Design review of the part shown in the three views and the two pictorial views. Dimensions are in mm from the part's minimum x, y and z. Give positions to 0.01 mm unless a question says otherwise; leave off trailing zeros. Order: outer loops, then holes, each group sorted by start corner. A loop starts at its lowest first (then second) coordinate and runs counter-clockwise, first axis right, second up. Notation, with made-up numbers: (88, -26) - (107, -26) arc R20 ccw to (107, -22) - close; hole circle Ø9 at (54.5, -26.75). An arc over 180 degrees is marked (long way). Put each result on its own line as item: value. Start each with the question number.
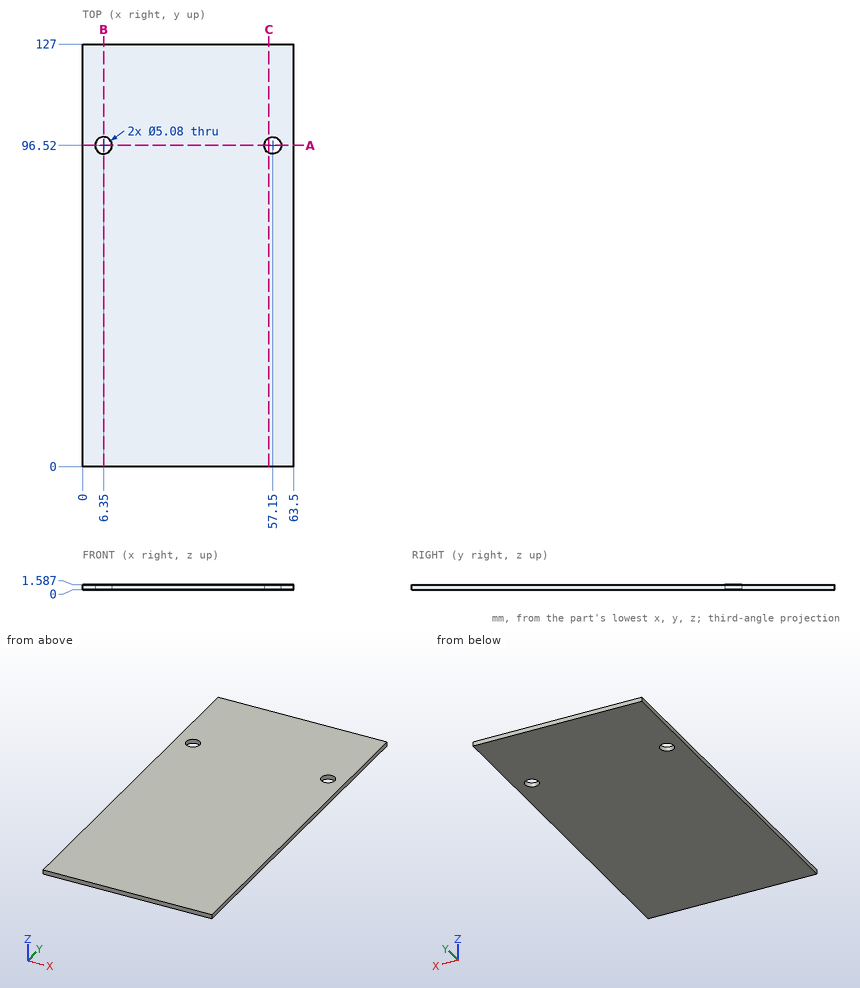
1. Add section C-C, the plane x = 56. Give the boundary of the cut face in (y, z) (1 decimal).
2. Wall thickness on line 1 (Y direction, x = 57.15, z = 0.9); line 2 (Y direction, x = 58.5, z = 1.2): over which ranges is each line inside the solid? List them lowest first. Write a range as from..to.
3. Add section A-A, the plane y = 96.52. Give the boundary of the cut face in (x, z).
4. Add section B-B, the plane x = 6.35. Give the boundary of the cut face in (y, z).
Found:
1. outline: (0, 0) - (94.3, 0) - (94.3, 1.6) - (0, 1.6) - close; (98.8, 0) - (127, 0) - (127, 1.6) - (98.8, 1.6) - close
2. line 1: y = 0..93.98, 99.06..127
2. line 2: y = 0..94.37, 98.67..127
3. outline: (0, 0) - (3.81, 0) - (3.81, 1.59) - (0, 1.59) - close; (8.89, 0) - (54.61, 0) - (54.61, 1.59) - (8.89, 1.59) - close; (59.69, 0) - (63.5, 0) - (63.5, 1.59) - (59.69, 1.59) - close
4. outline: (0, 0) - (93.98, 0) - (93.98, 1.59) - (0, 1.59) - close; (99.06, 0) - (127, 0) - (127, 1.59) - (99.06, 1.59) - close
